```python
from build123d import *

# Parameters (mm, degrees)
SKETCH1_W           = 180
SKETCH1_H           = 40
SKETCH1_W_2         = 170
SKETCH1_H_2         = 30
BOSS_EXTRUDE1_DEPTH = 90
FILLET1_R           = 1
SKETCH2_W           = 110
SKETCH2_H           = 50
CUT_EXTRUDE1_DEPTH  = 25
SKETCH3_W           = 50
SKETCH3_H           = 30
CUT_EXTRUDE2_DEPTH  = 16
SKETCH4_R           = 2.5
CUT_EXTRUDE3_DEPTH  = 1


with BuildPart() as part:
    # Sketch1 → Boss-Extrude1 (new body)
    with BuildSketch(Plane.XY):
        Rectangle(SKETCH1_W, SKETCH1_H)
        Rectangle(SKETCH1_W_2, SKETCH1_H_2, mode=Mode.SUBTRACT)
    extrude(amount=BOSS_EXTRUDE1_DEPTH)

    # Fillet1
    fillet1_edges = [part.edges().sort_by_distance(p)[0] for p in [
        (-90, 0, 90),
        (85, -15, 45),
        (85, 15, 45),
        (-85, 15, 45),
        (-85, -15, 45),
        (0, -20, 90),
        (90, 0, 90),
        (0, -20, 0),
        (-90, 0, 0),
        (0, 20, 0),
        (90, 0, 0),
        (90, -20, 45),
        (-90, -20, 45),
        (-90, 20, 45),
        (90, 20, 45),
        (0, 20, 90),
    ]]
    fillet(fillet1_edges, radius=FILLET1_R)

    # Sketch2 → Cut-Extrude1 (cut)
    with BuildSketch(Plane.XZ.offset(20)):
        with Locations((-34, 45)):
            Rectangle(SKETCH2_W, SKETCH2_H)
    extrude(amount=-CUT_EXTRUDE1_DEPTH, mode=Mode.SUBTRACT)

    # Sketch3 → Cut-Extrude2 (cut)
    with BuildSketch(Plane.ZY.offset(90)):
        with Locations((45, -5)):
            Rectangle(SKETCH3_W, SKETCH3_H)
    extrude(amount=-CUT_EXTRUDE2_DEPTH, mode=Mode.SUBTRACT)

    # Sketch4 → Cut-Extrude3 (cut)
    with BuildSketch(Plane.ZY.offset(90)):
        with Locations((10, -6.59211648)):
            Circle(SKETCH4_R)
        with Locations(Location((80, -6.59211648, 0), (0, 0, 180))):
            Circle(SKETCH4_R)
    extrude(amount=-CUT_EXTRUDE3_DEPTH, mode=Mode.SUBTRACT)


solid = part.part
```
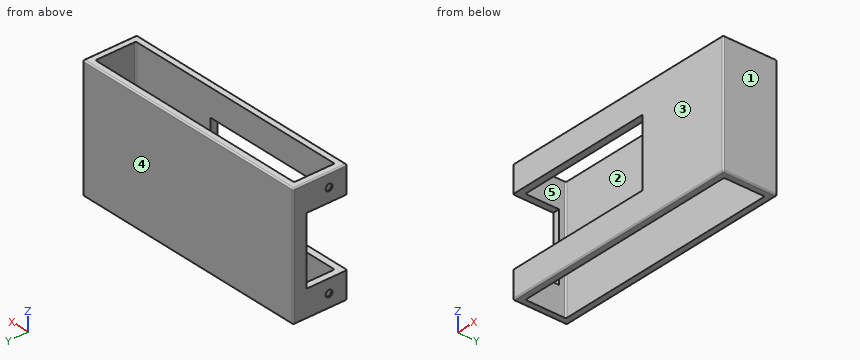
Could you check a few things on this model? Use its own coordinates, in mm. Face numbers are marked on the shaded views. A direction names the side the tool comes from. Round coordinates to 2 decimals unless told otherwise and drop trailing zeros. Loops run counter-clockwise (first coordinate to the right, second up) from the corner with the lowest first, then second, coordinate; pieces in that order, holes last. Notation, with made-up numbers: (-39, 20.25) - (-34, 20.25) arc R18 ccw to (-34, 28.25) - close; hole circle Ø8 at (67.5, 38.25). An arc over 180 degrees is marked (long way). Answer in a Markdown table with one row per item. Add a question column.
(1) If we section it at B-B (x = 60): Please give me the cut outline in (y, z), plus the area to 3 significant figures.
(2) If we mould it in two halves opening along Y, with no side actions, what happens to the marked faces 1, 2 and 3? For each: pulls with the +Y half, pulls with the -Y half, needs draft (parallel to the pull), parting line crosses it, or undercut.
(3) I need wall thicknesses on line 1 along X through (y, z) = (6.5, 17); line 2 along Y through (x, z) = (77.5, 67); line 3 along X through (y, z) = (-5.5, 46.5). Which ranges of each line are inside material? Lowest first, please.
(4) If we section it at D-D (z = 41): Please give me the cut outline in (x, y), plus the area to 3 significant figures.
(5) I'm going to push flat-ended pins straight in: pin 1 (5.5 mm diameter, centred on y = -16.5, z = 46.5, fed in from -X); pin 2 (1.5 mm diameter, centred on y = -7, z = 81, fed in from -X); pin 3 (2.5 mm diameter, centred on x = -87, z = 53, fed in from -Y); pin 4 (10 mm diameter, centred on x = 29, y = -7.5, fed in from -Z). Where does each tip first touch, or does it pass through?
(6) For the marked faces 4 and 5, which set-ups out of +Z, -Z, +X, -X, +Y, -Y let a thin tool reach every point of the face, with its end or its side?
(7) If we section it at C-C (x = -69): Please give me the cut outline in (y, z), plus the area to 3 significant figures.
(8) If we section it at A-A (y = 7): Please give me the cut outline in (x, z).
Model answer:
| question | item | result |
|---|---|---|
| 1 | outline | (-20, 1) arc R1 ccw to (-19, 0) - (-15, 0) - (-15, 90) - (-19, 90) arc R1 ccw to (-20, 89) - close; (15, 0) - (19, 0) arc R1 ccw to (20, 1) - (20, 89) arc R1 ccw to (19, 90) - (15, 90) - close |
| 1 | area | 899 mm² |
| 2 | face 1 | needs draft |
| 2 | face 2 | undercut |
| 2 | face 3 | pulls with the -Y half |
| 3 | line 1 | x = -90 to -85, 85 to 90 |
| 3 | line 2 | y = -20 to -15, 15 to 20 |
| 3 | line 3 | x = 85 to 90 |
| 4 | outline | (-90, 10) - (-85, 10) - (-85, 14) arc R1 cw to (-84, 15) - (84, 15) arc R1 cw to (85, 14) - (85, -14) arc R1 cw to (84, -15) - (21, -15) - (21, -20) - (89, -20) arc R1 ccw to (90, -19) - (90, 19) arc R1 ccw to (89, 20) - (-89, 20) arc R1 ccw to (-90, 19) - close |
| 4 | area | 1,420 mm² |
| 5 | pin 1 | stops at x = 21 |
| 5 | pin 2 | stops at x = -89 |
| 5 | pin 3 | stops at y = 10 |
| 5 | pin 4 | passes through |
| 6 | face 4 | +Z, -Z, +X, -X, +Y |
| 6 | face 5 | +Z, -Z |
| 7 | outline | (-20, 1) arc R1 ccw to (-19, 0) - (-15, 0) - (-15, 20) - (-20, 20) - close; (-20, 70) - (-15, 70) - (-15, 90) - (-19, 90) arc R1 ccw to (-20, 89) - close; (15, 0) - (19, 0) arc R1 ccw to (20, 1) - (20, 89) arc R1 ccw to (19, 90) - (15, 90) - close |
| 7 | area | 649 mm² |
| 8 | outline | (-90, 1) arc R1 ccw to (-89, 0) - (-85, 0) - (-85, 20) - (-90, 20) - close; (-90, 70) - (-85, 70) - (-85, 90) - (-89, 90) arc R1 ccw to (-90, 89) - close; (85, 0) - (89, 0) arc R1 ccw to (90, 1) - (90, 89) arc R1 ccw to (89, 90) - (85, 90) - close |
